Part model, mm, in its own coordinate system. Face numbers are marked on the shaded views. A direction names the side the tool comes from. Coordinates: 2 decimals unless noted, no trailing zeros. Write each loop counter-clockwise with the first axis right and the second up, starting at its lowest first coordinate (ties: lowest second). Pieces come first, ordered by that corner, then holes. Notation, with made-up numbers: (11, 39.5) -> (50, 39.5) arc R15 cw to (50, 59.5) -> close; hole circle Ø2 at (-36.5, -21.75). An arc over 180 degrees is marked (long way). Write item = value, one per line. Start each with the question number.
Q1. Probe line 1 (X direction, y = -25, z = -11.5); line 2 (Z direction, x = -31.5, y = -15); line 3 (Y direction, x = 21, z = -7). List the from-to ranges inside material, lowest first.
Q2. Band-saw the part on B-B, the plane y = -38. List the corners of the cut face in (x, z), plus the area to 3 significant figures.
Q3. Band-saw the part on C-C, the plane z = -27.5. List the corners of the cut face in (x, y), plus the area to 3 significant figures.
Q4. Pull direction X, two halves, no side cores. Call the marked faces 1, 2, 3 and 4: released by +X, released by -X, zero draft, split by the parting line, or undercut.
Q5. Band-saw the part on A-A, the plane x = -8.5. List the corners of the cut face in (y, z), plus the area to 3 significant figures.
Q6. Band-saw the part on D-D, the plane y = -12. List the corners of the cut face in (x, z), plus the area to 3 significant figures.
Q7. Tool access for the marked faces 5 and 6: list every direction of +Z, -Z, +X, -X, +Y, -Y with a clear straight run to the whole face (end or side of a thin tool).
Q8. Pin check, flat tips, straight feed: P1, Ø8, axis at x = 15.29, y = -24.43, coming from the -Z side; P2, Ø12, axis at x = -27, z = -19.5, coming from the +Y side; P3, Ø5, axis at x = -7.5, y = -34.5, coming from the -Z side. Stop position of each tip, or through.
from build123d import *

# Parameters (mm, degrees)
CROQUIS1_W              = 60
CROQUIS1_H              = 39
CROQUIS1_R              = 6
SALIENTE_EXTRUIR1_DEPTH = 4.7625
SALIENTE_EXTRUIR2_DEPTH = 4.7625
SALIENTE_EXTRUIR3_START = -60
SALIENTE_EXTRUIR3_DEPTH = 4.7625
CROQUIS4_W              = 60
CROQUIS4_H              = 4.7625
SALIENTE_EXTRUIR4_DEPTH = 25
CROQUIS5_R              = 3.5
CORTAR_EXTRUIR1_DEPTH   = 10


with BuildPart() as part:
    # Croquis1 → Saliente-Extruir1 (new body)
    with BuildSketch(Plane.XY):
        with Locations((-7.709348333, -11.433962264)):
            Rectangle(CROQUIS1_W, CROQUIS1_H)
        with Locations(Location((-7.709348333, -8.933962264, 0), (0, 0, 180))):
            Circle(CROQUIS1_R, mode=Mode.SUBTRACT)
    extrude(amount=SALIENTE_EXTRUIR1_DEPTH)

    # Croquis2 → Saliente-Extruir2 (add)
    with BuildSketch(Plane(origin=(22.290651667, 0, 0), x_dir=(0, 0, -1), z_dir=(1, 0, 0))):
        Polygon((-4.7625, 8.066037736), (-4.7625, -51.433962264), (34.352341017, -51.433962264), (0, 8.066037736), align=None)
    extrude(amount=SALIENTE_EXTRUIR2_DEPTH)

    # Croquis2<2> → Saliente-Extruir3 (add)
    with BuildSketch(Plane(origin=(22.290651667, 0, 0), x_dir=(0, 0, -1), z_dir=(1, 0, 0)).offset(SALIENTE_EXTRUIR3_START)):
        Polygon((-4.7625, 8.066037736), (-4.7625, -51.433962264), (34.352341017, -51.433962264), (0, 8.066037736), align=None)
    extrude(amount=-SALIENTE_EXTRUIR3_DEPTH)

    # Croquis4 → Saliente-Extruir4 (add)
    with BuildSketch(Plane.XY.offset(4.7625)):
        with Locations((-7.709348333, -33.315212264)):
            Rectangle(CROQUIS4_W, CROQUIS4_H)
    extrude(amount=-SALIENTE_EXTRUIR4_DEPTH)

    # Croquis5 → Cortar-Extruir1 (cut)
    with BuildSketch(Plane.XY.offset(4.7625)):
        with Locations((-30.709348333, -9.433962264)):
            Circle(CROQUIS5_R)
        with Locations((15.290651667, -9.433962264)):
            Circle(CROQUIS5_R)
        with Locations((15.290651667, -24.433962264)):
            Circle(CROQUIS5_R)
        with Locations((-30.709348333, -24.433962264)):
            Circle(CROQUIS5_R)
    extrude(amount=-CORTAR_EXTRUIR1_DEPTH, mode=Mode.SUBTRACT)


solid = part.part
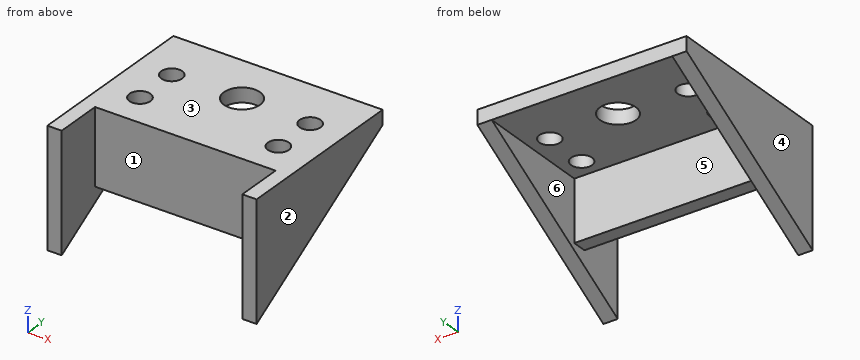
Ans:
q1.line_1 = -42.47 to -37.71, 22.29 to 27.05
q1.line_2 = 0 to 4.76
q1.line_3 = -35.7 to -30.93
q2.outline = (-42.47, -26.6) -> (-37.71, -26.6) -> (-37.71, 4.76) -> (-42.47, 4.76) -> close; (22.29, -26.6) -> (27.05, -26.6) -> (27.05, 4.76) -> (22.29, 4.76) -> close
q2.area = 299 mm2
q3.outline = (-42.47, -51.43) -> (-37.71, -51.43) -> (-37.71, -39.57) -> (-42.47, -39.57) -> close; (22.29, -51.43) -> (27.05, -51.43) -> (27.05, -39.57) -> (22.29, -39.57) -> close
q3.area = 113 mm2
q4.face_1 = undercut
q4.face_2 = released by +X
q4.face_3 = zero draft
q4.face_4 = released by -X
q5.outline = (-35.7, -20.24) -> (-30.93, -20.24) -> (-30.93, 0) -> (-14.88, 0) -> (-14.88, 4.76) -> (-35.7, 4.76) -> close; (-2.99, 0) -> (8.07, 0) -> (8.07, 4.76) -> (-2.99, 4.76) -> close
q5.area = 248 mm2
q6.outline = (-42.47, -11.59) -> (-37.71, -11.59) -> (-37.71, 0) -> (-33.09, 0) -> (-33.09, 4.76) -> (-42.47, 4.76) -> close; (-28.33, 0) -> (-12.87, 0) -> (-12.87, 4.76) -> (-28.33, 4.76) -> close; (-2.55, 0) -> (12.91, 0) -> (12.91, 4.76) -> (-2.55, 4.76) -> close; (17.67, 0) -> (22.29, 0) -> (22.29, -11.59) -> (27.05, -11.59) -> (27.05, 4.76) -> (17.67, 4.76) -> close
q6.area = 347 mm2
q7.face_5 = -Z, +Y
q7.face_6 = -Z
q8.P1 = 0
q8.P2 = -30.93
q8.P3 = -20.24
